Read the model definition and answer for the solid it produces. Units are mm, in the model's axes. Coordinates: 2 decimals unless noted, no trailing zeros. Write each loop counter-clockwise with the first axis right and the second up, starting at its lowest first coordinate (ties: lowest second). Pieces come first, ordered by that corner, then holes. Notation, with made-up numbers: M 66.5,26.5 L 116.5,26.5 A30 cw 116.5,55.5 Z; hole C -24,71.5 d7. An arc over 180 degrees is marked long. Write item = value, one per line.
Autodesk Inventor part; units mm, degrees
ref_plane "YZ Plane" through (0, 0, 0) normal (1, 0, 0) x (0, 1, 0)
ref_plane "XZ Plane" through (0, 0, 0) normal (0, 1, 0) x (-1, 0, 0)
ref_plane "XY Plane" through (0, 0, 0) normal (0, 0, 1) x (1, 0, 0)
ref_plane "Plano de trabajo5" through (0, 0, 0) normal (0, 0, 1) x (1, 0, 0)
sketch "Boceto2" plane through (0, 0, 0) normal (0, 0, 1) x (1, 0, 0)
  line L0 (0, 0) -> (20, 0)
  line L1 (20, 0) -> (20, -20)
  line L2 (20, -20) -> (0, -20)
  line L3 (0, -20) -> (0, 0)
  line L4 (0, -20) -> (6, -20)
  line L5 (6, -20) -> (6, -15)
  line L6 (6, -15) -> (6, -5)
  circle A0 centre (6, -15) radius 1.5
  circle A1 centre (6, -5) radius 1.5
  line L7 (20, -20) -> (20, -15)
  line L8 (20, -15) -> (16, -15)
  line L9 (16, -15) -> (16, -5)
  circle A2 centre (16, -15) radius 1.5
  circle A3 centre (16, -5) radius 1.5
  dimension "d17" = 20
  dimension "d18" = 20
  dimension "d19" = 6
  dimension "d20" = 5
  dimension "d21" = 10
  dimension "d22" = 3
  dimension "d23" = 3
  dimension "d24" = 5
  dimension "d25" = 4
  dimension "d26" = 10
  dimension "d27" = 3
  dimension "d28" = 3
extrude "Extrusión2" add sketch "Boceto2" along normal blind 3
fillet "Empalme2" radius 2 4 edges at (0, -20, 1.5) (0, 0, 1.5) (20, 0, 1.5) (20, -20, 1.5)
properties part number "Union 4"
Item 1: Find section B-B (y = -5). Determine the outline of the cut face in (x, z).
Worked answers:
outline = M 0,0 L 4.5,0 L 4.5,3 L 0,3 Z; M 7.5,0 L 14.5,0 L 14.5,3 L 7.5,3 Z; M 17.5,0 L 20,0 L 20,3 L 17.5,3 Z
Item 2: Find section A-A (x = 6). Determine the outline of the cut face in (y, z).
Worked answers:
outline = M -20,0 L -16.5,0 L -16.5,3 L -20,3 Z; M -13.5,0 L -6.5,0 L -6.5,3 L -13.5,3 Z; M -3.5,0 L 0,0 L 0,3 L -3.5,3 Z
Item 3: Consider line 1 along Y through (x, z) = (16, 2.15); line 2 along X through (y, z) = (-15, 2); line 3 along X through (y, z) = (-4.25, 1.15). Determine where each line is inside the solid, lowest interval first. Write a range as from..to.
Worked answers:
line_1 = -20..-16.5, -13.5..-6.5, -3.5..0
line_2 = 0..4.5, 7.5..14.5, 17.5..20
line_3 = 0..4.7, 7.3..14.7, 17.3..20
Item 4: Find section C-C (z = 2.4). Determine the outline of the cut face in (x, y).
Worked answers:
outline = M 0,-18 A2 ccw 2,-20 L 18,-20 A2 ccw 20,-18 L 20,-2 A2 ccw 18,0 L 2,0 A2 ccw 0,-2 Z; hole C 6,-15 d3; hole C 6,-5 d3; hole C 16,-15 d3; hole C 16,-5 d3
Item 5: For a pull along Y with two mould halves and no side action, classify faces 1 (the face through (10, -10, 3)), 2 (the face through (10, -20, 1)), 3 (the face through (4.89, -16.01, 1.48)) as released by +Y, released by -Y, zero draft, split by the parting line, or undercut.
Worked answers:
face_1 = zero draft
face_2 = released by -Y
face_3 = undercut
